Could you check a few things on this model? Use its own coordinates, in mm. A direction names the side the tool comes from. Give positions to 0.01 mm unless a question says otherwise; leave off trailing zeros. Loops run counter-clockwise (first coordinate to the right, second up) from the corner with the lowest first, then second, coordinate; pieces in that order, holes last. Notation, with made-up numbers: (-3, 20.25) -> (47, 20.25) arc R30 cw to (47, 44.25) -> close; hole circle Ø7 at (-16.5, -30.75). An arc over 180 degrees is marked (long way). Write item = value, one per line. Start each with the question number.
1) I need wall thicknesses on probe 1 along Z at (x, y) = (-51.5, 17); probe 2 along Z at (x, y) = (-65, 19.5); probe 3 along Y at (x, z) = (-67.25, 7.25). Which ranges of each line are inside material? Lowest first, please. Write a range as from..to.
2) I want a section at B-B (y = 18). List the corners of the cut face in (x, z) for me.
3) I want a section at C-C (x = -65). List the corners of the cut face in (y, z) for me, and give its area (3 significant figures).
4) On a 3-axis mill with a long thin cutter (end or side, diameter ignored), from which of +Z, -Z, +X, -X, +Y, -Y can I reach the whole of each face in a straight line? I mean faces 1 (the face through (-52, 27, 10)), 2 (the face through (-67, 28, 10)), 3 (the face through (-59.625, 16.418, 4.93)). Say none if no direction works.
5) I want a section at A-A (y = 4.25). List the corners of the cut face in (x, z) for me.
6) I want a section at D-D (z = 6.75). List the corners of the cut face in (x, y) for me.
7) I'm going to push flat-ended pins straight in: pin 1 Ø1.5 at (x, z) = (-64.5, 9.5) entering from +Y; pin 2 Ø12 at (x, z) = (-52, 21.5) entering from +Y; pin 3 Ø1.5 at (x, y) = (-70, 9) entering from -Z. Where does each tip first touch, or does it pass through?
from build123d import *

# Parameters (mm, degrees)
BOSS_EXTRUDE1_DEPTH = 10
BOSS_EXTRUDE2_DEPTH = 15


with BuildPart() as part:
    # Sketch1 → Boss-Extrude1 (new body)
    with BuildSketch(Plane.XY):
        with BuildLine():
            Line((-74.025675485, 30.818815331), (-44.815154686, 1.608294532))
            ThreePointArc((-44.815154686, 1.608294532), (-53.594607127, 22.03936289), (-74.025675485, 30.818815331))
        make_face()
    extrude(amount=BOSS_EXTRUDE1_DEPTH)

    # Sketch3 → Boss-Extrude2 (add)
    with BuildSketch(Plane.XY.offset(10)):
        with BuildLine():
            Line((-74.025675485, 1.608294532), (-44.815154686, 30.818815331))
            ThreePointArc((-44.815154686, 30.818815331), (-65.470112025, 22.263251871), (-74.025675485, 1.608294532))
        make_face()
    extrude(amount=BOSS_EXTRUDE2_DEPTH)


solid = part.part
Answer list:
q1.probe_1 = 0..10
q1.probe_2 = 10..25
q1.probe_3 = 24.04..29.86
q2.outline = (-68.99, 10) -> (-61.21, 10) -> (-61.21, 0) -> (-50.21, 0) -> (-50.21, 10) -> (-57.63, 10) -> (-57.63, 25) -> (-68.99, 25) -> close
q3.outline = (10.63, 10) -> (21.79, 10) -> (21.79, 0) -> (29.18, 0) -> (29.18, 10) -> (22.72, 10) -> (22.72, 25) -> (10.63, 25) -> close
q3.area = 255 mm^2
q4.face_1 = -Z, +X, +Y
q4.face_2 = +Z, -X, +Y
q4.face_3 = -Z, -X, -Y
q5.outline = (-73.91, 10) -> (-71.38, 10) -> (-71.38, 25) -> (-73.91, 25) -> close; (-47.46, 0) -> (-45, 0) -> (-45, 10) -> (-47.46, 10) -> close
q6.outline = (-74.03, 30.82) -> (-44.82, 1.61) arc R30.01 ccw to start
q7.pin_1 = 29.26
q7.pin_2 = 30.79
q7.pin_3 = 10
